Can you work these out from the model? Positions are in its coordinate system, mm. A direction names the side the tool comes from. Round coordinates to 2 decimals unless told otherwise and drop trailing zeros. Order: outer loops, then holes, each group sorted by start corner. A loop starts at its lowest first (then second) coordinate and runs counter-clockwise, first axis right, second up.
Q1. If we section it at C-C (x = 11.5): Please give me the cut outline in (y, z), plus the area to 3 significant figures.
Q2. If we section it at D-D (x = -1.5): Please give me the cut outline in (y, z).
Q3. If I drill on line 1 (X direction, y = 10, z = -13.5); line 2 (Y direction, x = 27.5, z = -9.5), over which ranges is the centre line in solid material (lowest first)?
Q4. For faces 4 (the face through (15, -1, -2.5)), 5 (the face through (0, -1, -6)), 6 (the face through (-9, 18, -14)), 7 (the face through (30, -1, -22)), which set-ups out of +Z, -Z, +X, -X, +Y, -Y let a thin tool reach every point of the face, with its end or its side?
Q5. We'd pull the mould along Y, two halves only. Please class faces 1 (the face through (-11, 35, -14)), 2 (the face through (41, 37, -14)), 3 (the face through (-10, 18, -13)): pulls with the +Y half, pulls with the -Y half, needs draft (parallel to the pull), parting line crosses it, or undercut.
Q6. If we section it at A-A (z = -22): Please give me the cut outline in (x, y).
Q7. If we section it at B-B (y = 18): Please give me the cut outline in (x, z).
Q8. Will these pins go through, and if not, where does the flat tip stop? P1, Ø2, axis at x = 6, z = -22.5, coming from the +Y side; P2, Ø1, axis at x = 34.5, y = -1.5, coming from the +Z side; P3, Ø1.6, axis at y = -0.5, z = -6, coming from the +X side; P4, Ø6, axis at x = 34, y = 33, coming from the -Z side.
Autodesk Inventor part; units mm, degrees
ref_plane "YZ Plane" through (0, 0, 0) normal (1, 0, 0) x (0, 1, 0)
ref_plane "XZ Plane" through (0, 0, 0) normal (0, 1, 0) x (-1, 0, 0)
ref_plane "XY Plane" through (0, 0, 0) normal (0, 0, 1) x (1, 0, 0)
sketch "Sketch2" plane through (0, 0, 0) normal (0, 1, 0) x (-1, 0, 0)
  line L0 (0, 0) -> (-30, 0)
  line L1 (-30, 0) -> (-30, -30)
  line L2 (-30, -30) -> (0, -30)
  line L3 (0, -30) -> (0, 0)
  line L4 (0, 0) -> (-30, 0)
  line L5 (-30, 0) -> (-30, -2)
  line L6 (0, -2) -> (0, 0)
  line L7 (0, -30) -> (-30, -30)
  line L8 (-30, -30) -> (-30, -44)
  line L9 (0, -44) -> (0, -30)
  point P0 (0, 0)
  dimension "d0" = 30
  dimension "d1" = 30
extrude "Extrusion2" add sketch "Sketch2" against normal blind 2
sketch "Sketch5" plane through (0, 0, 0) normal (0, 1, 0) x (1, 0, 0)
  line L0 (13.4, 2.5) -> (16.6, 2.5)
  line L1 (16.6, 2.5) -> (16.6, 27.5)
  line L2 (16.6, 27.5) -> (13.4, 27.5)
  line L3 (13.4, 27.5) -> (13.4, 2.5)
  line L4 (30, 30) -> (0, 30)
  line L5 (0, 30) -> (0, 0)
  line L6 (30, 0) -> (30, 30)
  point P0 (15, 2.5)
  point P1 (15, 27.5)
  dimension "d21" = 25
  dimension "d25" = 3.2
  dimension "d26" = 2.5
  dimension "d56" = 15
extrude "Extrusion5" cut sketch "Sketch5" against normal through all
sketch "Sketch6" plane through (0, 0, -30) normal (-1, 0, 0) x (0, 0, 1)
  line L0 (30, 0) -> (0, 0)
  line L1 (0, -2) -> (30, -2)
  line L2 (15, 0) -> (19, 0)
  line L3 (19, 0) -> (19, -2)
  line L4 (19, -2) -> (15, -2)
  line L5 (15, -2) -> (15, 0)
  line L6 (0, 0) -> (0, -2)
  point P0 (0, -1)
  point P1 (15, -1)
  point P2 (15, 0)
  dimension "d28" = 15
  dimension "d29" = 4
  dimension "d30" = 2
extrude "Extrusion6" add sketch "Sketch6" along normal blind 14 contours L3 L1 L5 L0
sketch "Sketch7" plane through (30, 0, 0) normal (1, 0, 0) x (0, 0, -1)
  line L0 (0, 0) -> (30, 0)
  line L1 (30, -2) -> (0, -2)
  line L2 (11, 0) -> (15, 0)
  line L3 (15, 0) -> (15, -2)
  line L4 (15, -2) -> (11, -2)
  line L5 (11, -2) -> (11, 0)
  line L6 (30, 0) -> (30, -2)
  point P0 (30, -1)
  point P1 (15, -1)
  point P2 (15, -2)
  dimension "d33" = 15
  dimension "d34" = 4
extrude "Extrusion7" add sketch "Sketch7" along normal blind 14 contours L0 L3 L1 L5
sketch "Sketch8" plane through (0, 0, 0) normal (0, 1, 0) x (1, 0, 0)
  line L0 (-14, 15) -> (-14, 11)
  line L1 (-14, 15) -> (-9, 15)
  line L2 (-9, 15) -> (-9, 13)
  line L3 (-9, 13) -> (-14, 13)
  line L4 (-14, 13) -> (-14, 15)
  line L5 (30, 15) -> (44, 15)
  line L6 (44, 15) -> (39, 15)
  line L7 (39, 15) -> (39, 13)
  line L8 (39, 13) -> (44, 13)
  line L9 (44, 13) -> (44, 15)
  point P0 (0, 0)
  point P1 (39, 15)
  point P2 (-14, 13)
  dimension "d37" = 5
  dimension "d38" = 2
  dimension "d39" = 5
  dimension "d40" = 2
extrude "Extrusion8" add sketch "Sketch8" along normal blind 37
sketch "Sketch9" plane through (-14, 0, -13) normal (0, 0, 1) x (1, 0, 0)
  line L0 (3.6, 35) -> (1.4, 35)
  line L1 (1.4, 35) -> (1.4, 2)
  line L2 (1.4, 2) -> (3.6, 2)
  line L3 (3.6, 2) -> (3.6, 35)
  line L4 (0, 37) -> (5, 37)
  line L5 (14, 0) -> (0, 0)
  line L6 (5, 0) -> (5, 37)
  line L7 (0, 0) -> (0, 37)
  line L8 (58, 0) -> (58, 37)
  line L9 (53, 0) -> (53, 37)
  line L10 (54.4, 35) -> (56.6, 35)
  line L11 (56.6, 35) -> (56.6, 2)
  line L12 (56.6, 2) -> (54.4, 2)
  line L13 (54.4, 2) -> (54.4, 35)
  line L14 (53, 37) -> (58, 37)
  line L15 (44, 0) -> (58, 0)
  point P0 (2.5, 37)
  point P1 (2.5, 35)
  point P2 (2.5, 2)
  point P3 (5, 18.5)
  point P4 (3.6, 18.5)
  point P5 (0, 18.5)
  point P6 (1.4, 18.5)
  point P7 (55.5, 37)
  point P8 (55.5, 35)
  point P9 (55.5, 2)
  dimension "d43" = 2
  dimension "d44" = 2
  dimension "d45" = 1.4
  dimension "d46" = 1.4
  dimension "d47" = 2.2
  dimension "d50" = 1.4
  dimension "d51" = 1.4
  dimension "d52" = 2
  dimension "d53" = 2
extrude "Extrusion9" cut sketch "Sketch9" against normal through all contours L3 L2 L1 L0 | L10 L11 L12 L13
properties part number "bobbin_support"
Solution:
1. outline: (-2, -30) - (0, -30) - (0, 0) - (-2, 0) - close
1. area: 60.0 mm2
2. outline: (-2, -15) - (0, -15) - (0, -11) - (-2, -11) - close
3. line 1: x = -14 to -12.6, -10.4 to -9, 39 to 40.4, 42.6 to 44
3. line 2: y = -2 to 0
4. face 4: +Y, -Y
4. face 5: +Z, -X, +Y, -Y
4. face 6: +Z, -Z, +Y
4. face 7: -Z, +X, +Y, -Y
5. face 1: undercut
5. face 2: pulls with the +Y half
5. face 3: needs draft
6. outline: (0, -2) - (13.4, -2) - (13.4, 0) - (0, 0) - close; (16.6, -2) - (30, -2) - (30, 0) - (16.6, 0) - close
7. outline: (-14, -15) - (-12.6, -15) - (-12.6, -13) - (-14, -13) - close; (-10.4, -15) - (-9, -15) - (-9, -13) - (-10.4, -13) - close; (39, -15) - (40.4, -15) - (40.4, -13) - (39, -13) - close; (42.6, -15) - (44, -15) - (44, -13) - (42.6, -13) - close
8. P1: stops at y = 0
8. P2: stops at z = -11
8. P3: stops at x = 30
8. P4: passes through
